```python
from build123d import *

# Parameters (mm, degrees)
BOSS_EXTRUDE1_DEPTH = 6.35
CUT_EXTRUDE2_DEPTH  = 12.7
CUT_EXTRUDE3_DEPTH  = 12.7
CHAMFER2_SIZE       = 1.5875


with BuildPart() as part:
    # Sketch1 → Boss-Extrude1 (new body)
    with BuildSketch(Plane.XY):
        with BuildLine():
            Line((0, 0), (12.7, 0))
            ThreePointArc((12.7, 0), (57.601280605, 18.598719395), (76.2, 63.5))
            Line((76.2, 63.5), (76.2, 76.2))
            Line((76.2, 76.2), (88.9, 76.2))
            Line((88.9, 76.2), (88.9, 63.5))
            ThreePointArc((88.9, 63.5), (66.581536726, 9.618463274), (12.7, -12.7))
            Line((12.7, -12.7), (0, -12.7))
            Line((0, -12.7), (0, 0))
        make_face()
    extrude(amount=BOSS_EXTRUDE1_DEPTH)

    # Sketch2 → Cut-Extrude2 (cut)
    with BuildSketch(Plane(origin=(0, 76.2, 0), x_dir=(1, 0, 0), z_dir=(0, 1, 0))):
        with BuildLine():
            Line((79.375, -1.5875), (85.725, -1.5875))
            ThreePointArc((85.725, -1.5875), (87.3125, -3.175), (85.725, -4.7625))
            Line((85.725, -4.7625), (79.375, -4.7625))
            ThreePointArc((79.375, -4.7625), (77.7875, -3.175), (79.375, -1.5875))
        make_face()
    extrude(amount=-CUT_EXTRUDE2_DEPTH, mode=Mode.SUBTRACT)

    # Sketch4 → Cut-Extrude3 (cut)
    with BuildSketch(Plane.ZY):
        with BuildLine():
            Line((4.7625, -3.175), (4.7625, -9.525))
            ThreePointArc((4.7625, -9.525), (3.175, -11.1125), (1.5875, -9.525))
            Line((1.5875, -9.525), (1.5875, -3.175))
            ThreePointArc((1.5875, -3.175), (3.175, -1.5875), (4.7625, -3.175))
        make_face()
    extrude(amount=-CUT_EXTRUDE3_DEPTH, mode=Mode.SUBTRACT)

    # Chamfer2
    chamfer2_edges = [part.edges().sort_by_distance(p)[0] for p in [
        (66.581536726, 9.618463274, 6.35),
        (6.35, -12.7, 0),
        (88.9, 69.85, 6.35),
        (76.2, 69.85, 6.35),
        (57.601280605, 18.598719395, 6.35),
        (6.35, 0, 6.35),
        (6.35, -12.7, 6.35),
        (6.35, 0, 0),
        (57.601280605, 18.598719395, 0),
        (76.2, 69.85, 0),
        (88.9, 69.85, 0),
        (66.581536726, 9.618463274, 0),
    ]]
    chamfer(chamfer2_edges, length=CHAMFER2_SIZE)


solid = part.part
```
The listing builds one solid part. Answer for the finished solid, in the listing's coordinates (mm). A direction names the side the tool comes from. Round coordinates to 2 decimals unless told otherwise and drop trailing zeros. Write each loop counter-clockwise with the first axis right and the second up, starting at its lowest first coordinate (ties: lowest second). Pieces come first, ordered by that corner, then holes. Notation, with made-up numbers: (46, 8.5) -> (66, 8.5) arc R13 ccw to (66, 29.5) -> close; hole circle Ø5 at (64.25, 16). An arc over 180 degrees is marked (long way). Write item = value, one per line.
1) Section B-B on z = 3.75 is taken. Write down the section's boundary in (x, y), plus the area to 3 significant figures.
Check values:
outline = (0, -12.7) -> (12.7, -12.7) arc R76.2 ccw to (88.9, 63.5) -> (88.9, 76.2) -> (87.2, 76.2) -> (87.2, 63.5) -> (77.9, 63.5) -> (77.9, 76.2) -> (76.2, 76.2) -> (76.2, 63.5) arc R63.5 cw to (12.7, 0) -> (0, 0) -> (0, -1.7) -> (12.7, -1.7) -> (12.7, -11) -> (0, -11) -> close
area = 1,480 mm²
2) Given pin 1 (1.6 mm diameter, centred on x = 81, z = 3, fed in from +Y); pin 2 (1 mm diameter, centred on x = 48.5, z = 3, fed in from -Y); pin 3 (3.5 mm diameter, centred on x = 5.5, z = 3, fed in from +Y), each flat-ended and moving along its own axis, determine where each tip first touches the part or whether it passes through.
Check values:
pin_1 = 63.5
pin_2 = -4.03
pin_3 = 0
3) Which of the six approach directions +Z, -Z, +X, -X, +Y, -Y give full straight-line access (tool end or side, diameter ignored) to faces 4 (the flat face through (76.2, 70, 3)), 5 (the flat face through (12.7, -6, 3)), 6 (the cylindrical face through (77.788, 69.939, 3.21)), 7 (the conical face through (66.233, 11.131, 0.276))?
Check values:
face_4 = +Z, -Z, -X, +Y
face_5 = -X
face_6 = +Y
face_7 = -Z, +X, -Y
4) For a pull along Z with two mould halves and no side action, classify faces 1 (the cylindrical face through (87.312, 69.939, 3.14)), 2 (the conical face through (57.3, 17.9, 1.3)), 3 (the flat face through (0, -6, 1)) as released by +Z, released by -Z, zero draft, split by the parting line, or undercut.
Check values:
face_1 = undercut
face_2 = released by -Z
face_3 = zero draft
5) Straight lines are drawn through the part: line 1 along X through (y, z) = (43.5, 4.5); line 2 along X through (y, z) = (66.5, 1.5); line 3 along Y through (x, z) = (51.5, 3.75). For each, find the intervals that lie inside material, in ascending order. Write a range as [from, to].
Check values:
line_1 = [72.97, 86.23]
line_2 = [76.29, 88.81]
line_3 = [-2.08, 13.23]
